Geometry: final body of the model. Coordinates: model frame, mm. Give positions to 0.01 mm unless a question says otherwise; leave off trailing zeros. Write each loop counter-clockwise with the first axis right and the second up, starting at its lowest first coordinate (ties: lowest second). Pieces come first, ordered by that corner, then holes.
Q1. Section D-D (z = -15). Return the cut outline in (x, y), plus the area to 3 significant figures.
Q2. Section B-B (y = 63.5). Return the cut outline in (x, z).
Q3. Line query: line 1 (Y direction, x = 3.75, z = -38.1); line 2 (Z direction, x = 5.5, y = 39); line 3 (Z direction, x = 1.75, y = 61). Output: solid intervals per line, ascending.
Q4. Section A-A (z = -38.1). Return the cut outline in (x, y), plus the area to 3 significant figures.
Q5. Mould query, pull axis Z, two halves, no side actions, for faces 1 (the cylindrical face through (3.22, 1.81, -48.89)), 2 (the cylindrical face through (3.131, 13.68, -41.213)), 3 (the flat face through (3, 0, -25)), 4 (the cylindrical face through (3.22, 74.29, -1.81)). Classes: +Z half, -Z half, draft (parallel to the pull), parting line (faces both ways), or undercut.
Q6. Pin query (flat end, axial travel): pin 1 Ø5 at (y, z) = (12.7, -38.1) entering from +X. Return the tip coordinate at first contact, or that it passes through.
Q7. Section C-C (x = 1.5). Return the cut outline in (y, z), plus the area to 3 significant figures.
from build123d import *

# Parameters (mm, degrees)
SKETCH1_W      = 50.8
SKETCH1_H      = 76.2
SKETCH1_R      = 3.2639
EXTRUDE1_DEPTH = 6.35
FILLET1_R      = 6.35


with BuildPart() as part:
    # Sketch1 → Extrude1 (new body)
    with BuildSketch(Plane(origin=(0, 0, 0), x_dir=(0, 0, -1), z_dir=(1, 0, 0))):
        with Locations((25.4, 38.1)):
            Rectangle(SKETCH1_W, SKETCH1_H)
        with Locations((12.7, 63.5)):
            Circle(SKETCH1_R, mode=Mode.SUBTRACT)
        with Locations((38.1, 63.5)):
            Circle(SKETCH1_R, mode=Mode.SUBTRACT)
        with Locations((12.7, 38.1)):
            Circle(SKETCH1_R, mode=Mode.SUBTRACT)
        with Locations((38.1, 38.1)):
            Circle(SKETCH1_R, mode=Mode.SUBTRACT)
        with Locations((12.7, 12.7)):
            Circle(SKETCH1_R, mode=Mode.SUBTRACT)
        with Locations((38.1, 12.7)):
            Circle(SKETCH1_R, mode=Mode.SUBTRACT)
    extrude(amount=EXTRUDE1_DEPTH)

    # Fillet1
    fillet1_edges = [part.edges().sort_by_distance(p)[0] for p in [
        (3.175, 76.2, 0),
        (3.175, 76.2, -50.8),
        (3.175, 0, -50.8),
        (3.175, 0, 0),
    ]]
    fillet(fillet1_edges, radius=FILLET1_R)


solid = part.part
Computed:
1. outline: (0, 0) - (6.35, 0) - (6.35, 10.38) - (0, 10.38) - close; (0, 15.02) - (6.35, 15.02) - (6.35, 35.78) - (0, 35.78) - close; (0, 40.42) - (6.35, 40.42) - (6.35, 61.18) - (0, 61.18) - close; (0, 65.82) - (6.35, 65.82) - (6.35, 76.2) - (0, 76.2) - close
1. area: 396 mm2
2. outline: (0, -50.8) - (6.35, -50.8) - (6.35, -41.36) - (0, -41.36) - close; (0, -34.84) - (6.35, -34.84) - (6.35, -15.96) - (0, -15.96) - close; (0, -9.44) - (6.35, -9.44) - (6.35, 0) - (0, 0) - close
3. line 1: y = 0 to 9.44, 15.96 to 34.84, 41.36 to 60.24, 66.76 to 76.2
3. line 2: z = -50.8 to -41.24, -34.96 to -15.84, -9.56 to 0
3. line 3: z = -50.8 to -40.2, -36 to -14.8, -10.6 to 0
4. outline: (0, 0) - (6.35, 0) - (6.35, 9.44) - (0, 9.44) - close; (0, 15.96) - (6.35, 15.96) - (6.35, 34.84) - (0, 34.84) - close; (0, 41.36) - (6.35, 41.36) - (6.35, 60.24) - (0, 60.24) - close; (0, 66.76) - (6.35, 66.76) - (6.35, 76.2) - (0, 76.2) - close
4. area: 360 mm2
5. face 1: -Z half
5. face 2: undercut
5. face 3: draft
5. face 4: +Z half
6. pin 1: passes through
7. outline: (0, -44.45) arc R6.35 ccw to (6.35, -50.8) - (69.85, -50.8) arc R6.35 ccw to (76.2, -44.45) - (76.2, -6.35) arc R6.35 ccw to (69.85, 0) - (6.35, 0) arc R6.35 ccw to (0, -6.35) - close; hole circle Ø6.53 at (12.7, -38.1); hole circle Ø6.53 at (12.7, -12.7); hole circle Ø6.53 at (38.1, -38.1); hole circle Ø6.53 at (38.1, -12.7); hole circle Ø6.53 at (63.5, -38.1); hole circle Ø6.53 at (63.5, -12.7)
7. area: 3,640 mm2
